Design review of the part built by this model. Coordinates are the model's own, in mm. A direction names the side the tool comes from. Coordinates: 2 decimals unless noted, no trailing zeros. Loops run counter-clockwise (first coordinate to the right, second up) from the corner with the lowest first, then second, coordinate; pieces in that order, holes last. Notation, with made-up numbers: (85.25, 59) -> (94.25, 59) arc R32 ccw to (94.25, 95) -> close; hole circle Ø8 at (34, 37.5). An arc over 180 degrees is marked (long way). Use one line per item in the form item = value. Start each with the question number.
1. Consider section C-C (y = 2). State the section outline as (x, z) points.
2. Machinability: for faces 1 (the face through (-42.47, 2.54, 1.61)), 2 (the face through (81, 10, 5)), which of the approach directions +Z, -Z, +X, -X, +Y, -Y give a long, thin tool a straight path to every point of the face, cutting with its end or side? Answer none if there is none.
3. Consider section B-B (x = -45). State the section outline as (y, z) points.
4. The part is to be moulded in two halves that separate along X. For faces 3 (the face through (110.95, 17.54, -0.78)), 4 (the face through (112.5, 17.46, -0.16)), 5 (the face through (2, 0, 0)), 6 (the face through (-107.93, 17.54, -0.65)), say which applies: released by +X, released by -X, zero draft, split by the parting line, or undercut.
5. Consider section D-D (x = 1). State the section outline as (y, z) points.
6. Consider section A-A (z = 0). State how many separate pieces and enclosed holes the cut face has, then the cut area to 3 significant figures.
7. For pin 1 (7 mm diameter, centred on x = 105, z = 0, fed in from +Y); pin 2 (3 mm diameter, centred on y = 10, z = -6.5, fed in from +X); pin 3 (1 mm diameter, centred on y = 15, z = -1, fed in from -X), all flat-tipped, find the tip position at first contact; note any pin that passes through.
8. Wall thickness on line 1 (Y direction, x = 15.5, z = 1.75); line 2 (Z direction, x = -85.5, y = 8); line 3 (X direction, y = 4, z = 0.75): over which ranges is each line inside the solid? List them lowest first. Write a range as from..to.
from build123d import *

# Parameters (mm, degrees)
EXTRUDE_1_DEPTH     = 20
SKETCH_2_W          = 150
SKETCH_2_H          = 10
CUT_EXTRUDE_3_DEPTH = 116.244305716
SKETCH_3_W          = 25
SKETCH_3_H          = 10
CUT_EXTRUDE_4_DEPTH = 116.244305716
SKETCH_4_W          = 10
SKETCH_4_H          = 10
CUT_EXTRUDE_5_DEPTH = 202.137390855
SKETCH_5_R          = 3
SKETCH_5_R_2        = 6
CUT_EXTRUDE_6_DEPTH = 115.509824906
SKETCH_6_R          = 3
CUT_EXTRUDE_7_DEPTH = 115.509824906


with BuildPart() as part:
    # 草图1 → 凸台-拉伸1 (new body)
    with BuildSketch(Plane(origin=(0, 0, 0), x_dir=(1, 0, 0), z_dir=(0, 1, 0))):
        with BuildLine():
            Line((-105, 7.5), (105, 7.5))
            ThreePointArc((105, 7.5), (112.5, 0), (105, -7.5))
            Line((105, -7.5), (-105, -7.5))
            ThreePointArc((-105, -7.5), (-112.5, 0), (-105, 7.5))
        make_face()
    extrude(amount=EXTRUDE_1_DEPTH)

    # 草图2 → 切除-拉伸3 (cut, through all)
    with BuildSketch(Plane(origin=(0, 0, -7.5), x_dir=(-1, 0, 0), z_dir=(0, 0, -1))):
        with Locations((0, 10)):
            Rectangle(SKETCH_2_W, SKETCH_2_H)
    extrude(amount=-CUT_EXTRUDE_3_DEPTH, mode=Mode.SUBTRACT)

    # 草图3 → 切除-拉伸4 (cut, through all)
    with BuildSketch(Plane(origin=(0, 0, -7.5), x_dir=(-1, 0, 0), z_dir=(0, 0, -1))):
        with Locations((100, 10)):
            Rectangle(SKETCH_3_W, SKETCH_3_H)
        with Locations((-100, 10)):
            Rectangle(SKETCH_3_W, SKETCH_3_H)
    extrude(amount=-CUT_EXTRUDE_4_DEPTH, mode=Mode.SUBTRACT)

    # 草图4 → 切除-拉伸5 (cut, through all)
    with BuildSketch(Plane.ZY.offset(87.5)):
        with Locations((0, 10)):
            Rectangle(SKETCH_4_W, SKETCH_4_H)
    extrude(amount=-CUT_EXTRUDE_5_DEPTH, mode=Mode.SUBTRACT)

    # 草图5 → 切除-拉伸6 (cut, through all)
    with BuildSketch(Plane(origin=(0, 20, 0), x_dir=(1, 0, 0), z_dir=(0, 1, 0))):
        with Locations(Location((-105, 0, 0), (0, 0, 270))):
            Circle(SKETCH_5_R)
        with Locations(Location((105, 0, 0), (0, 0, 270))):
            Circle(SKETCH_5_R_2)
    extrude(amount=-CUT_EXTRUDE_6_DEPTH, mode=Mode.SUBTRACT)

    # 草图6 → 切除-拉伸7 (cut, through all)
    with BuildSketch(Plane(origin=(0, 20, 0), x_dir=(1, 0, 0), z_dir=(0, 1, 0))):
        with Locations(Location((-45, 0, 0), (0, 0, 270))):
            Circle(SKETCH_6_R)
    extrude(amount=-CUT_EXTRUDE_7_DEPTH, mode=Mode.SUBTRACT)


solid = part.part
Geometry check:
q1.outline = (-105, -7.5) -> (105, -7.5) arc R7.5 ccw to (105, 7.5) -> (-105, 7.5) arc R7.5 ccw to start; hole circle Ø6 at (-105, 0); hole circle Ø6 at (-45, 0); hole circle Ø12 at (105, 0)
q2.face_1 = +Y, -Y
q2.face_2 = +X, -X
q3.outline = (0, -7.5) -> (5, -7.5) -> (5, -3) -> (0, -3) -> close; (0, 3) -> (5, 3) -> (5, 7.5) -> (0, 7.5) -> close; (15, -7.5) -> (20, -7.5) -> (20, -3) -> (15, -3) -> close; (15, 3) -> (20, 3) -> (20, 7.5) -> (15, 7.5) -> close
q4.face_3 = undercut
q4.face_4 = released by +X
q4.face_5 = zero draft
q4.face_6 = undercut
q5.outline = (0, -7.5) -> (5, -7.5) -> (5, 7.5) -> (0, 7.5) -> close; (15, -7.5) -> (20, -7.5) -> (20, 7.5) -> (15, 7.5) -> close
q6.separate_pieces = 8
q6.enclosed_holes = 0
q6.area = 2,010 mm²
q7.pin_1 = through
q7.pin_2 = 87.5
q7.pin_3 = -112.48
q8.line_1 = 0..5, 15..20
q8.line_2 = -7.5..-5, 5..7.5
q8.line_3 = -112.46..-107.9, -102.1..-47.9, -42.1..99.05, 110.95..112.46
